```python
from build123d import *

# Parameters (mm, degrees)
SKETCH1_R           = 12
SKETCH1_R_2         = 1.2
SKETCH1_R_3         = 2.075
BOSS_EXTRUDE1_DEPTH = 5
CUT_EXTRUDE1_DEPTH  = 5


with BuildPart() as part:
    # Sketch1 → Boss-Extrude1 (new body)
    with BuildSketch(Plane(origin=(0, 0, 0), x_dir=(1, 0, 0), z_dir=(0, 1, 0))):
        with BuildLine():
            Line((-134.118891506, 0), (134.118891506, 0))
            ThreePointArc((134.118891506, 0), (137.928249972, 1.76136015), (139.053747558, 5.804484769))
            Line((139.053747558, 5.804484769), (120.84297072, 117.512705691))
            ThreePointArc((120.84297072, 117.512705691), (119.443648574, 120.243754828), (116.712599437, 121.643076974))
            Line((116.712599437, 121.643076974), (84.336583334, 126.921044874))
            ThreePointArc((84.336583334, 126.921044874), (81.605534197, 128.32036702), (80.206212051, 131.051416157))
            Line((80.206212051, 131.051416157), (60.683956749, 250.804484769))
            ThreePointArc((60.683956749, 250.804484769), (58.987740546, 253.809358466), (55.749100697, 255))
            Line((55.749100697, 255), (-55.749100697, 255))
            ThreePointArc((-55.749100697, 255), (-58.987740546, 253.809358466), (-60.683956749, 250.804484769))
            Line((-60.683956749, 250.804484769), (-80.206212051, 131.051416157))
            ThreePointArc((-80.206212051, 131.051416157), (-81.605534197, 128.32036702), (-84.336583334, 126.921044874))
            Line((-84.336583334, 126.921044874), (-116.712599437, 121.643076974))
            ThreePointArc((-116.712599437, 121.643076974), (-119.443648574, 120.243754828), (-120.84297072, 117.512705691))
            Line((-120.84297072, 117.512705691), (-139.053747558, 5.804484769))
            ThreePointArc((-139.053747558, 5.804484769), (-137.928249972, 1.76136015), (-134.118891506, 0))
        make_face()
        with Locations((0, 195)):
            Circle(SKETCH1_R, mode=Mode.SUBTRACT)
        with Locations((-70, 60)):
            Circle(SKETCH1_R, mode=Mode.SUBTRACT)
        with Locations((70, 60)):
            Circle(SKETCH1_R, mode=Mode.SUBTRACT)
        with Locations((-22.5, 82.5)):
            Circle(SKETCH1_R_2, mode=Mode.SUBTRACT)
        with Locations((22.5, 82.5)):
            Circle(SKETCH1_R_2, mode=Mode.SUBTRACT)
        with Locations((22.5, 37.5)):
            Circle(SKETCH1_R_2, mode=Mode.SUBTRACT)
        with Locations((-22.5, 37.5)):
            Circle(SKETCH1_R_2, mode=Mode.SUBTRACT)
        with Locations((-50.091827035, 135.325391796)):
            Circle(SKETCH1_R_3, mode=Mode.SUBTRACT)
        with Locations((50.091827035, 135.325391796)):
            Circle(SKETCH1_R_3, mode=Mode.SUBTRACT)
        with Locations((0, 17)):
            Circle(SKETCH1_R_3, mode=Mode.SUBTRACT)
        with BuildLine():
            Line((12.5, 127.5), (-12.5, 127.5))
            ThreePointArc((-12.5, 127.5), (-20, 135), (-12.5, 142.5))
            Line((-12.5, 142.5), (12.5, 142.5))
            ThreePointArc((12.5, 142.5), (20, 135), (12.5, 127.5))
        make_face(mode=Mode.SUBTRACT)
        with BuildLine():
            Line((12.5, 97.5), (-12.5, 97.5))
            ThreePointArc((-12.5, 97.5), (-20, 105), (-12.5, 112.5))
            Line((-12.5, 112.5), (12.5, 112.5))
            ThreePointArc((12.5, 112.5), (20, 105), (12.5, 97.5))
        make_face(mode=Mode.SUBTRACT)
    extrude(amount=BOSS_EXTRUDE1_DEPTH)

    # Sketch2 → Cut-Extrude1 (cut)
    with BuildSketch(Plane(origin=(0, 5, 0), x_dir=(1, 0, 0), z_dir=(0, 1, 0))):
        Polygon((-60.578994825, 214.111244254), (-51.568858582, 242.831053531), (-46.559589522, 241.259518139), (-55.569725765, 212.539708863), align=None)
        Polygon((-118.431141418, 12.168946469), (-109.421005175, 40.888755746), (-114.430274235, 42.460291137), (-123.440410478, 13.740481861), align=None)
        Polygon((123.440410478, 13.740481861), (114.430274235, 42.460291137), (109.421005175, 40.888755746), (118.431141418, 12.168946469), align=None)
        Polygon((55.569725765, 212.539708863), (46.559589522, 241.259518139), (51.568858582, 242.831053531), (60.578994825, 214.111244254), align=None)
    extrude(amount=-CUT_EXTRUDE1_DEPTH, mode=Mode.SUBTRACT)


solid = part.part
```
Verification items for the finished model (mm, model axes). A direction names the side the tool comes from. Round coordinates to 2 decimals unless told otherwise and drop trailing zeros. Write each loop counter-clockwise with the first axis right and the second up, starting at its lowest first coordinate (ties: lowest second). Pieces come first, ordered by that corner, then holes.
1. Gauge pin test, flat ends, axial feed: P1, Ø1, axis at y = 3, z = -44, coming from the -X side; P2, Ø2, axis at x = -78, z = -123.5, coming from the -Y side. Record the tip position at first contact, or that the pin passes through.
2. Section check A-A on x = -68.5. Enter the section's corners in (y, z).
3. Draft check along X on faces 3 (the flat face through (-33, 0, -101)), 4 (the flat face through (113.863, 2.535, -26.73)), 5 (the flat face through (-70.308, 2.465, -191.766)). Enter one of: +X half, -X half, draft (parallel to the pull), parting line (faces both ways), or undercut.
4. Section check C-C on y = 2.1. State how many separate pieces and enclosed holes the cut face has, plus the area to 3 significant figures.
5. Scan lines: L1, parallel to Z at x = -22.5, y = 2.85; L2, parallel to Z at x = 0, y = 1.4 (3 decimals); L3, parallel to X at y = 3.75, z = -60. Record each from-to range of solid material in increasing order.
6. Access from +Z, -Z, +X, -X, +Y, -Y to the whole of each face (thin tool, end or side, straight path). Record for faces 1 (the flat face through (-129.82, 2.46, -62.44)), 2 (the flat face through (-118.872, 2.535, -28.301)).
7. Section check D-D on z = -179. Enter the section's corners in (x, y), plus the area to 3 significant figures.
8. Section check B-B on z = -24. Enter the section's corners in (x, y), plus the area to 3 significant figures.
Answer:
1. P1: stops at x = -132.91
1. P2: stops at y = 0
2. outline: (0, -202.86) - (5, -202.86) - (5, -71.91) - (0, -71.91) - close; (0, -48.09) - (5, -48.09) - (5, 0) - (0, 0) - close
3. face 3: draft
3. face 4: undercut
3. face 5: -X half
4. separate pieces: 1
4. enclosed holes: 16
4. area: 47,600 mm2
5. L1: z = -255 to -83.7, -81.3 to -38.7, -36.3 to 0
5. L2: z = -255 to -207, -183 to -142.5, -127.5 to -112.5, -97.5 to -19.075, -14.925 to 0
5. L3: x = -130.22 to -82, -58 to 58, 82 to 130.22
6. face 1: -Z, -X, +Y, -Y
6. face 2: +Y, -Y
7. outline: (-72.39, 0) - (72.39, 0) - (72.39, 5) - (-72.39, 5) - close
7. area: 724 mm2
8. outline: (-136.09, 0) - (-120.22, 0) - (-120.22, 5) - (-136.09, 5) - close; (-114.72, 0) - (114.72, 0) - (114.72, 5) - (-114.72, 5) - close; (120.22, 0) - (136.09, 0) - (136.09, 5) - (120.22, 5) - close
8. area: 1,310 mm2
